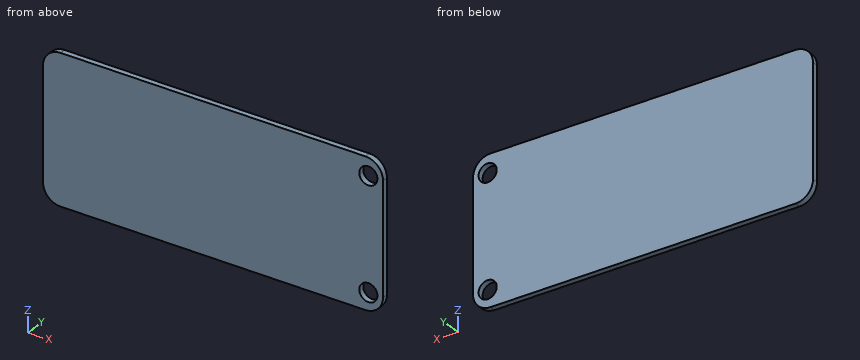
from build123d import *

# Parameters (mm, degrees)
SKETCH_1_W          = 58
SKETCH_1_H          = 25
EXTRUDE_1_DEPTH     = 1
SKETCH_2_R          = 1.55
CUT_EXTRUDE_1_DEPTH = 2
FILLET_1_R          = 3


with BuildPart() as part:
    # 草图1 → 凸台-拉伸1 (new body)
    with BuildSketch(Plane(origin=(0, 0, 0), x_dir=(1, 0, 0), z_dir=(0, 1, 0))):
        Rectangle(SKETCH_1_W, SKETCH_1_H)
    extrude(amount=EXTRUDE_1_DEPTH)

    # 草图2 → 切除-拉伸1 (cut, through all)
    with BuildSketch(Plane(origin=(0, 1, 0), x_dir=(1, 0, 0), z_dir=(0, 1, 0))):
        with Locations((26.5, 9.5)):
            Circle(SKETCH_2_R)
        with Locations((26.5, -9.5)):
            Circle(SKETCH_2_R)
    extrude(amount=-CUT_EXTRUDE_1_DEPTH, mode=Mode.SUBTRACT)

    # 圆角1
    fillet_1_edges = [part.edges().sort_by_distance(p)[0] for p in [
        (29, 0.5, 12.5),
        (-29, 0.5, 12.5),
        (-29, 0.5, -12.5),
        (29, 0.5, -12.5),
    ]]
    fillet(fillet_1_edges, radius=FILLET_1_R)


solid = part.part
Part model, mm, in its own coordinate system. Give positions to 0.01 mm unless a question says otherwise; leave off trailing zeros. Write each loop counter-clockwise with the first axis right and the second up, starting at its lowest first coordinate (ties: lowest second). Pieces come first, ordered by that corner, then holes.
1) Cut at A-A on y = 0.65. Write the cut outline in (x, z), then the cut area to 3 significant figures.
Resolved:
outline: (-29, -9.5) arc R3 ccw to (-26, -12.5) - (26, -12.5) arc R3 ccw to (29, -9.5) - (29, 9.5) arc R3 ccw to (26, 12.5) - (-26, 12.5) arc R3 ccw to (-29, 9.5) - close; hole circle Ø3.1 at (26.5, -9.5); hole circle Ø3.1 at (26.5, 9.5)
area: 1,430 mm2
2) Pin check, flat tips, straight feed: pin 1 (4 mm diameter, centred on x = 26.5, z = -9.5, fed in from -Y); pin 2 (1.9 mm diameter, centred on x = 26.5, z = 9.5, fed in from +Y). Stop position of each tip, or through.
Resolved:
pin 1: stops at y = 0
pin 2: passes through
3) Probe L1, parallel to Z at x = 26.5, y = 0.7; L2, parallel to X at y = 0.65, z = 9.5; L3, parallel to X at y = 0.65, z = -10.75. List the from-to ranges inside material, lowest first.
Resolved:
L1: z = -12.46 to -11.05, -7.95 to 7.95, 11.05 to 12.46
L2: x = -29 to 24.95, 28.05 to 29
L3: x = -28.73 to 25.58, 27.42 to 28.73
